from build123d import *

# Parameters (mm, degrees)
P_IDAT_VYSUNUT_M1_DEPTH                           = 17
V_LCOV_ZAHLOUBEN_PRO_M6_ROUBY_S_HLAVO_D           = 6.6
V_LCOV_ZAHLOUBEN_PRO_M6_ROUBY_S_HLAVO_CBORE_D     = 8.3
V_LCOV_ZAHLOUBEN_PRO_M6_ROUBY_S_HLAVO_CBORE_DEPTH = 10
V_LCOV_ZAHLOUBEN_PRO_M6_ROUBY_S_H_2_D             = 6.6
V_LCOV_ZAHLOUBEN_PRO_M6_ROUBY_S_H_2_CBORE_D       = 12
V_LCOV_ZAHLOUBEN_PRO_M6_ROUBY_S_H_2_CBORE_DEPTH   = 2
ZAOBLIT1_R                                        = 4
P_IDAT_VYSUNUT_M4_DEPTH                           = 3
ZKOSEN_1_SIZE                                     = 3


with BuildPart() as part:
    # Skica1 → Přidat vysunutím1 (new body)
    with BuildSketch(Plane.XY):
        with BuildLine():
            Line((0, 0), (50, 0))
            Line((50, 0), (50, -8))
            ThreePointArc((50, -8), (49.414213562, -9.414213562), (48, -10))
            Line((48, -10), (32.5, -10))
            Line((32.5, -10), (32.5, -22))
            Line((32.5, -22), (17.5, -22))
            Line((17.5, -22), (17.5, -10))
            Line((17.5, -10), (2, -10))
            ThreePointArc((2, -10), (0.585786438, -9.414213562), (0, -8))
            Line((0, -8), (0, 0))
        make_face()
    extrude(amount=P_IDAT_VYSUNUT_M1_DEPTH)

    # V_lcov_ zahlouben_ pro M6 _rouby s hlavo (through all)
    with Locations(Plane.XY.offset(17)):
        with Locations((25, -15)):
            CounterBoreHole(V_LCOV_ZAHLOUBEN_PRO_M6_ROUBY_S_HLAVO_D / 2, V_LCOV_ZAHLOUBEN_PRO_M6_ROUBY_S_HLAVO_CBORE_D / 2, V_LCOV_ZAHLOUBEN_PRO_M6_ROUBY_S_HLAVO_CBORE_DEPTH)

    # V_lcov_ zahlouben_ pro M6 _rouby s h 2 (through all)
    with Locations(Plane(origin=(0, -10, 0), x_dir=(-1, 0, 0), z_dir=(0, -1, 0))):
        with Locations((-9.5, -8.5), (-40.5, -8.5)):
            CounterBoreHole(V_LCOV_ZAHLOUBEN_PRO_M6_ROUBY_S_H_2_D / 2, V_LCOV_ZAHLOUBEN_PRO_M6_ROUBY_S_H_2_CBORE_D / 2, V_LCOV_ZAHLOUBEN_PRO_M6_ROUBY_S_H_2_CBORE_DEPTH)

    # Zaoblit1
    zaoblit1_edges = [part.edges().sort_by_distance(p)[0] for p in [
        (32.5, -22, 8.5),
        (17.5, -22, 8.5),
    ]]
    fillet(zaoblit1_edges, radius=ZAOBLIT1_R)

    # Skica10 → Přidat vysunutím4 (add)
    with BuildSketch(Plane(origin=(0, 0, 0), x_dir=(1, 0, 0), z_dir=(0, 1, 0))):
        with BuildLine():
            Line((15.75, -8.5), (34.25, -8.5))
            ThreePointArc((34.25, -8.5), (34.623047352, -6.373047352), (35.697656822, -4.5))
            Line((35.697656822, -4.5), (14.302343178, -4.5))
            ThreePointArc((14.302343178, -4.5), (15.376952648, -6.373047352), (15.75, -8.5))
        make_face()
        with BuildLine():
            ThreePointArc((35.697656822, -12.5), (34.623047352, -10.626952648), (34.25, -8.5))
            Line((34.25, -8.5), (15.75, -8.5))
            ThreePointArc((15.75, -8.5), (15.376952648, -10.626952648), (14.302343178, -12.5))
            Line((14.302343178, -12.5), (35.697656822, -12.5))
        make_face()
        with BuildLine():
            ThreePointArc((4.697656822, -12.5), (3.623047352, -10.626952648), (3.25, -8.5))
            Line((3.25, -8.5), (0, -8.5))
            Line((0, -8.5), (0, -12.5))
            Line((0, -12.5), (4.697656822, -12.5))
        make_face()
        with BuildLine():
            Line((0, -8.5), (3.25, -8.5))
            ThreePointArc((3.25, -8.5), (3.623047352, -6.373047352), (4.697656822, -4.5))
            Line((4.697656822, -4.5), (0, -4.5))
            Line((0, -4.5), (0, -8.5))
        make_face()
        with BuildLine():
            Line((46.75, -8.5), (50, -8.5))
            Line((50, -8.5), (50, -4.5))
            Line((50, -4.5), (45.302343178, -4.5))
            ThreePointArc((45.302343178, -4.5), (46.376952648, -6.373047352), (46.75, -8.5))
        make_face()
        with BuildLine():
            Line((50, -12.5), (50, -8.5))
            Line((50, -8.5), (46.75, -8.5))
            ThreePointArc((46.75, -8.5), (46.376952648, -10.626952648), (45.302343178, -12.5))
            Line((45.302343178, -12.5), (50, -12.5))
        make_face()
    extrude(amount=P_IDAT_VYSUNUT_M4_DEPTH)

    # Zkosení1
    zkosen_1_edges = [part.edges().sort_by_distance(p)[0] for p in [
        (25, 3, 4.5),
        (2.348828411, 3, 4.5),
        (47.651171589, 3, 4.5),
    ]]
    chamfer(zkosen_1_edges, length=ZKOSEN_1_SIZE - 0.0001)  # a hair under: the kernel refuses the full size


solid = part.part
Part model, mm, in its own coordinate system. A direction names the side the tool comes from. Round coordinates to 2 decimals unless told otherwise and drop trailing zeros. Write each loop counter-clockwise with the first axis right and the second up, starting at its lowest first coordinate (ties: lowest second). Pieces come first, ordered by that corner, then holes. Notation, with made-up numbers: (-37.5, 58) - (-31.5, 58) arc R37 ccw to (-31.5, 94) - close; hole circle Ø7 at (-39, 2). An arc over 180 degrees is marked (long way). Use CSV: the item, a comma, the result in double quotes.
Item 1: Slice it at A-A, the plane y = -15. Write the cut outline in (x, z).
Results list:
outline,"(17.5, 0) - (21.7, 0) - (21.7, 7) - (20.85, 7) - (20.85, 17) - (17.5, 17) - close; (28.3, 0) - (32.5, 0) - (32.5, 17) - (29.15, 17) - (29.15, 7) - (28.3, 7) - close"
Item 2: Slice it at C-C, the plane z = 1.25. Write the cut outline in (x, y).
Results list:
outline,"(0, -8) arc R2 ccw to (2, -10) - (17.5, -10) - (17.5, -18) arc R4 ccw to (21.5, -22) - (28.5, -22) arc R4 ccw to (32.5, -18) - (32.5, -10) - (48, -10) arc R2 ccw to (50, -8) - (50, 0) - (0, 0) - close; hole circle Ø6.6 at (25, -15)"
Item 3: Flat gauge pins, fed straight in: P1, Ø1.5, axis at x = 23.5, y = 2, coming from the +Z side; P2, Ø8.5, axis at x = 40.5, z = 8.5, coming from the +Y side; P3, Ø9.5, axis at x = 39, z = 8, coming from the -Y side. Where does each tip first touch, or does it go through?
Results list:
P1,"stops at z = 12.5"
P2,"stops at y = 0"
P3,"stops at y = -10"
Item 4: Tool access for faces 1 (the flat face through (22, -17, 7)), 2 (the flat face through (35, -10, 5)), 3 (the flat face through (17.5, -14, 8)), 4 (the flat face through (48, 1, 12.5)): list every direction of +Z, -Z, +X, -X, +Y, -Y with a clear straight run to the whole face (end or side of a thin tool).
Results list:
face 1,"+Z"
face 2,"+Z, -Z, +X, -Y"
face 3,"+Z, -Z, -X, -Y"
face 4,"+Z, +X, -X, +Y"
Item 5: Pull direction X, two halves, no side cores. Call faces 5 (the flat face through (7, -8, 11)), 6 (the flat face through (38, -8, 11)), 7 (the flat face through (2, 1, 12.5)), 8 (the flat face through (32.5, -14, 8)): pulls with the +X half, pulls with the -X half, needs draft (parallel to the pull), parting line crosses it, or undercut.
Results list:
face 5,"undercut"
face 6,"undercut"
face 7,"needs draft"
face 8,"pulls with the +X half"
Item 6: Slice it at B-B, the plane x = 9.5. Write the cut outline in (y, z).
Results list:
outline,"(-10, 0) - (0, 0) - (0, 5.2) - (-8, 5.2) - (-8, 2.5) - (-10, 2.5) - close; (-10, 14.5) - (-8, 14.5) - (-8, 11.8) - (0, 11.8) - (0, 17) - (-10, 17) - close"
Item 7: Wall check: L1, parallel to X at y = -5.75, z = 8.5; L2, parallel to Y at x = 25, z = 14.5; L3, parallel to Y at x = 25, z = 10.25. Give the ranges that are in metal, low to high.
Results list:
L1,"x = 0 to 6.2, 12.8 to 37.2, 43.8 to 50"
L2,"y = -22 to -19.15, -10.85 to 0"
L3,"y = -22 to -19.15, -10.85 to 3"
